from build123d import *

# Parameters (mm, degrees)
SKETCH1_R           = 95.25
BOSS_EXTRUDE1_DEPTH = 3.81
SKETCH2_R           = 95.25
SKETCH2_R_2         = 91.44
BOSS_EXTRUDE2_DEPTH = 13.97
HOLE1_OUTLINE_R     = 12.7
HOLE1_DEPTH         = 3.81


# Read off the part's stored shape, not the designer's step: Hole1
with BuildPart() as part:
    # Sketch1 → Boss-Extrude1 (new body)
    with BuildSketch(Plane(origin=(0, 0, 0), x_dir=(1, 0, 0), z_dir=(0, 1, 0))):
        with Locations(Location((0, 0, 0), (0, 0, 90))):
            Circle(SKETCH1_R)
    extrude(amount=BOSS_EXTRUDE1_DEPTH)

    # Sketch2 → Boss-Extrude2 (add)
    with BuildSketch(Plane(origin=(0, 3.81, 0), x_dir=(1, 0, 0), z_dir=(0, 1, 0))):
        with Locations(Location((0, 0, 0), (0, 0, 90))):
            Circle(SKETCH2_R)
        with Locations(Location((0, 0, 0), (0, 0, 270))):
            Circle(SKETCH2_R_2, mode=Mode.SUBTRACT)
    extrude(amount=BOSS_EXTRUDE2_DEPTH)

    # Hole1 outline → Hole1 (cut)
    with BuildSketch(Plane(origin=(0, 0, 0), x_dir=(1, 0, 0), z_dir=(0, 1, 0))):
        with Locations((-68.958152294, -11.126353047)):
            Circle(HOLE1_OUTLINE_R)
    extrude(amount=HOLE1_DEPTH, mode=Mode.SUBTRACT)


solid = part.part
Here's how the part is built. I have some questions about the finished solid (model axes, mm). A direction names the side the tool comes from. Coordinates: 2 decimals unless noted, no trailing zeros. Loops run counter-clockwise (first coordinate to the right, second up) from the corner with the lowest first, then second, coordinate; pieces in that order, holes last.
1. For P1, Ø3, axis at x = 38.5, y = 13.5, coming from the +Z side; P2, Ø1, axis at y = 8.5, z = 6, coming from the -X side; P3, Ø12, axis at x = -52, z = -56, coming from the +Y side, each with a flat end and sliding along its axis, tell me the tip position at first contact or that it passes through.
2. I need wall thicknesses on L1, parallel to X at y = 13.25, z = 0; L2, parallel to Y at x = -25.5, z = 58; L3, parallel to X at y = 13.5, z = -79. Which ranges of each line are inside material? Lowest first, please.
3. For faces 1 (the cylindrical face through (-56.845, 1.878, 7.312)), 2 (the flat face through (-1, 3.81, 1)), which set-ups out of +Z, -Z, +X, -X, +Y, -Y let a thin tool reach every point of the face, with its end or its side?
4. Imagine slicing it at A-A, the plane x = 0. Please give me the cut outline in (y, z).
5. Imagine slicing it at B-B, the plane y = 12. Please give me the cut outline in (x, z), and give its area (3 significant figures).
6. If we mould it in two halves opening along X, with no side actions, what happens to faces 3 (the flat face through (-1, 0, 1)), 4 (the cylindrical face through (90.662, 10.697, -11.904)), 5 (the cylindrical face through (92.985, 8.766, 20.648))? For each: pulls with the +X half, pulls with the -X half, needs draft (parallel to the pull), parting line crosses it, or undercut.
7. Imagine slicing it at C-C, the plane z = 72.5. Please give me the cut outline in (x, y), and give its area (3 significant figures).
Taken from the geometry:
1. P1: stops at z = 87.77
1. P2: stops at x = -95.09
1. P3: stops at y = 3.81
2. L1: x = -95.25 to -91.44, 91.44 to 95.25
2. L2: y = 0 to 3.81
2. L3: x = -53.21 to -46.05, 46.05 to 53.21
3. face 1: +Y, -Y
3. face 2: +Y
4. outline: (0, -95.25) - (17.78, -95.25) - (17.78, -91.44) - (3.81, -91.44) - (3.81, 91.44) - (17.78, 91.44) - (17.78, 95.25) - (0, 95.25) - close
5. outline: circle Ø190.5 at (0, 0); hole circle Ø182.88 at (0, 0)
5. area: 2,230 mm2
6. face 3: needs draft
6. face 4: undercut
6. face 5: parting line crosses it
7. outline: (-61.78, 0) - (61.78, 0) - (61.78, 17.78) - (55.72, 17.78) - (55.72, 3.81) - (-55.72, 3.81) - (-55.72, 17.78) - (-61.78, 17.78) - close
7. area: 640 mm2
